Can you work these out from the model? Positions are in its coordinate system, mm. A direction names the side the tool comes from. Coordinates: 2 decimals unless noted, no trailing zeros. Order: outer loops, then holes, each group sorted by start corner. A loop starts at its lowest first (then second) coordinate and runs counter-clockwise, first axis right, second up. Notation, with made-up numbers: (47.5, -37) -> (52.5, -37) arc R18 ccw to (52.5, -26) -> close; hole circle Ø2 at (46.25, -36.5). An arc over 180 degrees is marked (long way). Use a Markdown table: item, result. Add a question column.
1. We'd pull the mould along X, two halves only. Please class faces 3 (the cylindrical face through (78.865, 594.794, 739.5)), 4 (the cylindrical face through (132.107, 591.425, 760.5)), 5 (the flat face through (586, -137, 0)), 6 (the cylindrical face through (183.6, -576.5, 1114.6)): pulls with the +X half, pulls with the -X half, needs draft (parallel to the pull), parting line crosses it, or undercut.
2. If I drill on line 1 along Z through (x, y) = (0, -600.5); line 2 along Y through (x, z) = (-228, 1389); line 3 along Y through (x, z) = (-301, 120), over which ranges is the centre line in solid material (lowest first)? Write a range as from..to.
3. For faces 1 (the flat face through (586, -137, 1500)), 2 (the cylindrical face through (-36.95, -602.28, 1393.68)), which set-ups out of +Z, -Z, +X, -X, +Y, -Y let a thin tool reach every point of the face, with its end or its side?
4. Suppose I cut it at A-A, the plane x = 466.5. List the corners of the cut face in (y, z) for me, then the cut area to 3 significant figures.
5. Suppose I cut it at B-B, the plane z = 1048. List the corners of the cut face in (x, y) for me.
6. For pin 1 Ø6 at (y, z) = (-134, 668) entering from -X; pin 2 Ø3 at (x, z) = (123.5, 1016) entering from +Y; pin 3 Ø2 at (x, z) = (157, 614) entering from -Y, each with a flat end and sliding along its axis, tell me the tip position at first contact or that it passes through.
7. Suppose I cut it at D-D, the plane z = 443. List the corners of the cut face in (x, y) for me.
8. Suppose I cut it at C-C, the plane x = 7.5. List the corners of the cut face in (y, z) for me.
Autodesk Inventor part; units mm, degrees
ref_plane "YZ Plane" through (0, 0, 0) normal (1, 0, 0) x (0, 1, 0)
ref_plane "XZ Plane" through (0, 0, 0) normal (0, 1, 0) x (-1, 0, 0)
ref_plane "XY Plane" through (0, 0, 0) normal (0, 0, 1) x (1, 0, 0)
sketch "Sketch1" plane through (0, 0, 0) normal (0, 1, 0) x (-1, 0, 0)
  line L0 (606, 1500) -> (600, 1500)
  line L1 (600, 1500) -> (600, 0)
  line L2 (600, 0) -> (606, 0)
  line L3 (606, 0) -> (606, 1500)
  line L4 (0, 0) -> (0, 1673.0415)
  point P0 (603, 0)
  dimension "d0" = 6
  dimension "d1" = 1500
  dimension "d2" = 1200
revolve "Revolution1" add sketch "Sketch1" angle 359.9 about axis through (0, 0, 0) along (0, 0, 1)
sketch "Sketch2" plane through (0, 0, 0) normal (0, 1, 0) x (-1, 0, 0)
  circle A0 centre (0, 1019) radius 207
  circle A1 centre (0, 131) radius 40
  circle A2 centre (0, 1409) radius 40
  line L0 (600, 1500) -> (-600, 1500)
  point P0 (0, 0)
  point P1 (599.9991, 1500)
  dimension "d4" = 414
  dimension "d5" = 80
  dimension "d6" = 80
  dimension "d7" = 131
  dimension "d8" = 91
  dimension "d9" = 481
extrude "Extrusion1" cut sketch "Sketch2" against normal through all
equation "\"d1\" = Высота_сред_части"
equation "\"d2\" = Внутр_Диам"
equation "\"d4\" = Внутр_диам_ревиз_окна"
equation "\"d5\" = Внешний_диам_трубы_подкл"
equation "\"d6\" = Внешний_диам_трубы_подкл"
equation "\"BendRadius\" = Thickness"
equation "\"BendReliefWidth\" = Thickness"
equation "\"BendReliefDepth\" = 0.5 * Thickness"
equation "\"CornerReliefSize\" = 4 * Thickness"
equation "\"MinimumRemnant\" = 2 * Thickness"
equation "\"TransitionRadius\" = BendRadius"
equation "\"JacobiRadiusSize\" = BendRadius"
equation "\"GapSize\" = Thickness"
properties part number "Стенка фильтра D1200"
Worked out:
| question | item | result |
|---|---|---|
| 1 | face 3 | undercut |
| 1 | face 4 | parting line crosses it |
| 1 | face 5 | needs draft |
| 1 | face 6 | undercut |
| 2 | line 1 | z = 0..91, 171..812, 1226..1369, 1449..1500 |
| 2 | line 2 | y = -561.47..-554.99, 554.99..561.47 |
| 2 | line 3 | y = -525.96..-519.04, 519.04..525.96 |
| 3 | face 1 | +Z, +X, -X, +Y, -Y |
| 3 | face 2 | -Y |
| 4 | outline | (-386.8, 0) -> (-377.33, 0) -> (-377.33, 1500) -> (-386.8, 1500) -> close; (377.33, 0) -> (386.8, 0) -> (386.8, 1500) -> (377.33, 1500) -> close |
| 4 | area | 28,400 mm² |
| 5 | outline | (-606, 0) arc R606 ccw to (-204.96, -570.29) -> (-204.96, -563.91) arc R600 cw to (-600, 0) -> close; (-606, 1.06) -> (-600, 1.05) arc R600 cw (long way) to (204.96, -563.91) -> (204.96, -570.29) arc R606 ccw (long way) to start |
| 6 | pin 1 | stops at x = -591.67 |
| 6 | pin 2 | stops at y = 593.59 |
| 6 | pin 3 | stops at y = -585.58 |
| 7 | outline | (-606, 0) arc R606 ccw (long way) to (-606, 1.06) -> (-600, 1.05) arc R600 cw (long way) to (-600, 0) -> close |
| 8 | outline | (-605.95, 0) -> (-599.95, 0) -> (-599.95, 91.71) -> (-605.95, 91.71) -> close; (-605.95, 170.29) -> (-599.95, 170.29) -> (-599.95, 812.14) -> (-605.95, 812.14) -> close; (-605.95, 1225.86) -> (-599.95, 1225.86) -> (-599.95, 1369.71) -> (-605.95, 1369.71) -> close; (-605.95, 1448.29) -> (-599.95, 1448.29) -> (-599.95, 1500) -> (-605.95, 1500) -> close; (599.95, 0) -> (605.95, 0) -> (605.95, 1500) -> (599.95, 1500) -> close |
